```python
from build123d import *

# Parameters (mm, degrees)
SKETCH1_R           = 11.5
SKETCH1_R_2         = 1.75
BOSS_EXTRUDE1_DEPTH = 3.2
BOSS_EXTRUDE2_START = 3.2
SKETCH1_5_R         = 2.55
SKETCH1_5_R_2       = 11.5
SKETCH1_5_R_3       = 1.75
BOSS_EXTRUDE2_DEPTH = 3
BOSS_EXTRUDE3_START = 5
SKETCH1_6_R         = 2.55
BOSS_EXTRUDE3_DEPTH = 1.2
CUT_EXTRUDE2_START  = 3.2
SKETCH1_4_R         = 3
CUT_EXTRUDE2_DEPTH  = 3
FILLET1_R           = 3


with BuildPart() as part:
    # Sketch1 → Boss-Extrude1 (new body)
    with BuildSketch(Plane(origin=(0, -68.726755499, 0), x_dir=(1, 0, 0), z_dir=(0, 1, 0))):
        with BuildLine():
            Line((100.657671875, -32.65), (132.000817625, -32.65))
            ThreePointArc((132.000817625, -32.65), (132.689647804, -32.512983159), (133.273609832, -32.122792206))
            Line((133.273609832, -32.122792206), (136.602036956, -28.794365081))
            ThreePointArc((136.602036956, -28.794365081), (136.992227909, -28.210403054), (137.12924475, -27.521572875))
            Line((137.12924475, -27.521572875), (137.12924475, 3.821572875))
            ThreePointArc((137.12924475, 3.821572875), (136.992227909, 4.510403054), (136.602036956, 5.094365081))
            Line((136.602036956, 5.094365081), (133.273609832, 8.422792206))
            ThreePointArc((133.273609832, 8.422792206), (132.689647804, 8.812983159), (132.000817625, 8.95))
            Line((132.000817625, 8.95), (100.657671875, 8.95))
            ThreePointArc((100.657671875, 8.95), (99.968841697, 8.812983159), (99.384879669, 8.422792206))
            Line((99.384879669, 8.422792206), (96.056452544, 5.094365081))
            ThreePointArc((96.056452544, 5.094365081), (95.666261592, 4.510403054), (95.52924475, 3.821572875))
            Line((95.52924475, 3.821572875), (95.52924475, -27.521572875))
            ThreePointArc((95.52924475, -27.521572875), (95.666261592, -28.210403054), (96.056452544, -28.794365081))
            Line((96.056452544, -28.794365081), (99.384879669, -32.122792206))
            ThreePointArc((99.384879669, -32.122792206), (99.968841697, -32.512983159), (100.657671875, -32.65))
        make_face()
        with Locations((116.32924475, -11.85)):
            Circle(SKETCH1_R, mode=Mode.SUBTRACT)
        with Locations((100.82924475, -27.35)):
            Circle(SKETCH1_R_2, mode=Mode.SUBTRACT)
        with Locations((100.82924475, 3.65)):
            Circle(SKETCH1_R_2, mode=Mode.SUBTRACT)
        with Locations((131.82924475, 3.65)):
            Circle(SKETCH1_R_2, mode=Mode.SUBTRACT)
        with Locations((131.82924475, -27.35)):
            Circle(SKETCH1_R_2, mode=Mode.SUBTRACT)
    extrude(amount=BOSS_EXTRUDE1_DEPTH)

    # Sketch1<5> → Boss-Extrude2 (add)
    with BuildSketch(Plane(origin=(0, -68.726755499, 0), x_dir=(1, 0, 0), z_dir=(0, 1, 0)).offset(BOSS_EXTRUDE2_START)):
        with BuildLine():
            Line((108.32924475, 8.95), (100.657671875, 8.95))
            ThreePointArc((100.657671875, 8.95), (99.968841697, 8.812983159), (99.384879669, 8.422792206))
            Line((99.384879669, 8.422792206), (96.056452544, 5.094365081))
            ThreePointArc((96.056452544, 5.094365081), (95.666261592, 4.510403054), (95.52924475, 3.821572875))
            Line((95.52924475, 3.821572875), (95.52924475, -27.521572875))
            ThreePointArc((95.52924475, -27.521572875), (95.666261592, -28.210403054), (96.056452544, -28.794365081))
            Line((96.056452544, -28.794365081), (99.384879669, -32.122792206))
            ThreePointArc((99.384879669, -32.122792206), (99.968841697, -32.512983159), (100.657671875, -32.65))
            Line((100.657671875, -32.65), (156.32924475, -32.65))
            Line((156.32924475, -32.65), (156.32924475, 28))
            Line((156.32924475, 28), (108.32924475, 28))
            Line((108.32924475, 28), (108.32924475, 8.95))
        make_face()
        with Locations((144.32924475, -16)):
            Circle(SKETCH1_5_R, mode=Mode.SUBTRACT)
        with Locations((152.32924475, -16)):
            Circle(SKETCH1_5_R, mode=Mode.SUBTRACT)
        with Locations((144.32924475, -8)):
            Circle(SKETCH1_5_R, mode=Mode.SUBTRACT)
        with Locations((152.32924475, -8)):
            Circle(SKETCH1_5_R, mode=Mode.SUBTRACT)
        with Locations((120.32924475, 16)):
            Circle(SKETCH1_5_R, mode=Mode.SUBTRACT)
        with Locations((120.32924475, 24)):
            Circle(SKETCH1_5_R, mode=Mode.SUBTRACT)
        with Locations((144.32924475, 0)):
            Circle(SKETCH1_5_R, mode=Mode.SUBTRACT)
        with Locations((152.32924475, 0)):
            Circle(SKETCH1_5_R, mode=Mode.SUBTRACT)
        with Locations((144.32924475, 8)):
            Circle(SKETCH1_5_R, mode=Mode.SUBTRACT)
        with Locations((152.32924475, 8)):
            Circle(SKETCH1_5_R, mode=Mode.SUBTRACT)
        with Locations((128.32924475, 16)):
            Circle(SKETCH1_5_R, mode=Mode.SUBTRACT)
        with Locations((136.32924475, 16)):
            Circle(SKETCH1_5_R, mode=Mode.SUBTRACT)
        with Locations((128.32924475, 24)):
            Circle(SKETCH1_5_R, mode=Mode.SUBTRACT)
        with Locations((136.32924475, 24)):
            Circle(SKETCH1_5_R, mode=Mode.SUBTRACT)
        with Locations((144.32924475, 16)):
            Circle(SKETCH1_5_R, mode=Mode.SUBTRACT)
        with Locations((152.32924475, 16)):
            Circle(SKETCH1_5_R, mode=Mode.SUBTRACT)
        with Locations((144.32924475, 24)):
            Circle(SKETCH1_5_R, mode=Mode.SUBTRACT)
        with Locations((152.32924475, 24)):
            Circle(SKETCH1_5_R, mode=Mode.SUBTRACT)
        with Locations((116.32924475, -11.85)):
            Circle(SKETCH1_5_R_2, mode=Mode.SUBTRACT)
        with Locations((112.32924475, 24)):
            Circle(SKETCH1_5_R, mode=Mode.SUBTRACT)
        with Locations((112.32924475, 16)):
            Circle(SKETCH1_5_R, mode=Mode.SUBTRACT)
        with Locations((100.82924475, -27.35)):
            Circle(SKETCH1_5_R_3, mode=Mode.SUBTRACT)
        with Locations((100.82924475, 3.65)):
            Circle(SKETCH1_5_R_3, mode=Mode.SUBTRACT)
        with Locations((131.82924475, 3.65)):
            Circle(SKETCH1_5_R_3, mode=Mode.SUBTRACT)
        with Locations((131.82924475, -27.35)):
            Circle(SKETCH1_5_R_3, mode=Mode.SUBTRACT)
    extrude(amount=BOSS_EXTRUDE2_DEPTH)

    # Sketch1<6> → Boss-Extrude3 (add)
    with BuildSketch(Plane(origin=(0, -68.726755499, 0), x_dir=(1, 0, 0), z_dir=(0, 1, 0)).offset(BOSS_EXTRUDE3_START)):
        with Locations((152.32924475, -16)):
            Circle(SKETCH1_6_R)
        with Locations((144.32924475, -16)):
            Circle(SKETCH1_6_R)
        with Locations((144.32924475, -8)):
            Circle(SKETCH1_6_R)
        with Locations((152.32924475, -8)):
            Circle(SKETCH1_6_R)
        with Locations((152.32924475, 0)):
            Circle(SKETCH1_6_R)
        with Locations((144.32924475, 0)):
            Circle(SKETCH1_6_R)
        with Locations((152.32924475, 8)):
            Circle(SKETCH1_6_R)
        with Locations((152.32924475, 16)):
            Circle(SKETCH1_6_R)
        with Locations((144.32924475, 24)):
            Circle(SKETCH1_6_R)
        with Locations((152.32924475, 24)):
            Circle(SKETCH1_6_R)
        with Locations((136.32924475, 24)):
            Circle(SKETCH1_6_R)
        with Locations((136.32924475, 16)):
            Circle(SKETCH1_6_R)
        with Locations((128.32924475, 16)):
            Circle(SKETCH1_6_R)
        with Locations((128.32924475, 24)):
            Circle(SKETCH1_6_R)
        with Locations((120.32924475, 16)):
            Circle(SKETCH1_6_R)
        with Locations((120.32924475, 24)):
            Circle(SKETCH1_6_R)
        with Locations((144.32924475, 8)):
            Circle(SKETCH1_6_R)
        with Locations((144.32924475, 16)):
            Circle(SKETCH1_6_R)
        with Locations((112.32924475, 24)):
            Circle(SKETCH1_6_R)
        with Locations((112.32924475, 16)):
            Circle(SKETCH1_6_R)
    extrude(amount=BOSS_EXTRUDE3_DEPTH)

    # Sketch1<4> → Cut-Extrude2 (cut)
    with BuildSketch(Plane(origin=(0, -68.726755499, 0), x_dir=(1, 0, 0), z_dir=(0, 1, 0)).offset(CUT_EXTRUDE2_START)):
        with Locations((100.82924475, -27.35)):
            Circle(SKETCH1_4_R)
        with Locations((100.82924475, 3.65)):
            Circle(SKETCH1_4_R)
        with Locations((131.82924475, 3.65)):
            Circle(SKETCH1_4_R)
        with Locations((131.82924475, -27.35)):
            Circle(SKETCH1_4_R)
    extrude(amount=CUT_EXTRUDE2_DEPTH, mode=Mode.SUBTRACT)

    # Fillet1
    fillet1_edges = [part.edges().sort_by_distance(p)[0] for p in [
        (156.32924475, -64.026755499, 32.65),
        (108.32924475, -64.026755499, -8.95),
    ]]
    fillet(fillet1_edges, radius=FILLET1_R)


solid = part.part
```
Work out the finished part from the listing and answer in its coordinate system (mm). A direction names the side the tool comes from. Give positions to 0.01 mm unless a question says otherwise; leave off trailing zeros. Order: outer loops, then holes, each group sorted by start corner. A loop starts at its lowest first (then second) coordinate and runs counter-clockwise, first axis right, second up. Notation, with made-up numbers: (-13.5, -22) -> (33.5, -22) arc R37 ccw to (33.5, 14) -> close; hole circle Ø9 at (81, -2.5). An arc over 180 degrees is marked (long way). Answer as CSV lines item,"result". Start each with the question number.
(1) Section C-C, the plane x = 113.5 is taken. Write down the section's boundary in (y, z).
(2) Section B-B, the plane y = -67 is taken. Write down the section's boundary in (x, z).
(3) Consider line 1 along X through (y, z) = (-64.25, -9.5); line 2 along X through (y, z) = (-67, -4); line 3 along Y through (x, z) = (102, -2). Determine where each line is inside the solid, lowest interval first.
(4) Which of the six approach directions +Z, -Z, +X, -X, +Y, -Y give full straight-line access (tool end or side, diameter ignored) to faces 5 (the cylindrical face through (130.441, -67.149, 28.415)), 6 (the flat face through (144, -63.727, 16)), 7 (the flat face through (102, -65.527, -2))?
(5) Section A-A, the plane z = 11.85 is taken. Write down the section's boundary in (x, y), plus the area to 3 significant figures.
(6) Section D-D, the plane z = -24 is taken. Write down the section's boundary in (x, y).
(7) Each of these flat-tipped pins is pushed along its axis until it touches: pin 1 Ø5.5 at (x, z) = (136.5, -23) entering from -Y; pin 2 Ø2.5 at (x, z) = (144.5, 7) entering from -Y; pin 3 Ø1 at (x, y) = (102, -66.5) entering from -Z. Where does it stop, or does it pass through?
(8) For a pull along Z with two mould halves and no side action, classify faces 1 (the flat face through (121, -65, 32.65)), 2 (the flat face through (95.529, -66, 12)), 3 (the flat face through (133, -65.527, 29)), 4 (the cylindrical face through (109.78, -64.64, -16.11)) as released by +Z, released by -Z, zero draft, split by the parting line, or undercut.
Entries:
1,outline,"(-68.73, -8.95) -> (-65.53, -8.95) -> (-65.53, -13.73) -> (-63.73, -13.73) -> (-63.73, -18.27) -> (-65.53, -18.27) -> (-65.53, -21.73) -> (-63.73, -21.73) -> (-63.73, -26.27) -> (-65.53, -26.27) -> (-65.53, -28) -> (-62.53, -28) -> (-62.53, 0.7) -> (-68.73, 0.7) -> close; (-68.73, 23) -> (-62.53, 23) -> (-62.53, 32.65) -> (-68.73, 32.65) -> close"
2,outline,"(95.53, -3.82) arc R1.8 ccw to (96.06, -5.09) -> (99.38, -8.42) arc R1.8 ccw to (100.66, -8.95) -> (132, -8.95) arc R1.8 ccw to (133.27, -8.42) -> (136.6, -5.09) arc R1.8 ccw to (137.13, -3.82) -> (137.13, 27.52) arc R1.8 ccw to (136.6, 28.79) -> (133.27, 32.12) arc R1.8 ccw to (132, 32.65) -> (100.66, 32.65) arc R1.8 ccw to (99.38, 32.12) -> (96.06, 28.79) arc R1.8 ccw to (95.53, 27.52) -> close; hole circle Ø3.5 at (100.83, -3.65); hole circle Ø3.5 at (100.83, 27.35); hole circle Ø23 at (116.33, 11.85); hole circle Ø3.5 at (131.83, -3.65); hole circle Ø3.5 at (131.83, 27.35)"
3,line 1,"107.06 to 142.27, 146.39 to 150.27, 154.39 to 156.33"
3,line 2,"95.54 to 99.11, 102.54 to 130.11, 133.54 to 137.12"
3,line 3,"-68.73 to -65.53"
4,face 5,"+Y, -Y"
4,face 6,"-Y"
4,face 7,"+Y"
5,outline,"(95.53, -68.73) -> (104.83, -68.73) -> (104.83, -62.53) -> (95.53, -62.53) -> close; (127.83, -68.73) -> (137.13, -68.73) -> (137.13, -65.53) -> (156.33, -65.53) -> (156.33, -62.53) -> (127.83, -62.53) -> close"
5,area,"173 mm²"
6,outline,"(108.33, -65.53) -> (109.78, -65.53) -> (109.78, -63.73) -> (114.88, -63.73) -> (114.88, -65.53) -> (117.78, -65.53) -> (117.78, -63.73) -> (122.88, -63.73) -> (122.88, -65.53) -> (125.78, -65.53) -> (125.78, -63.73) -> (130.88, -63.73) -> (130.88, -65.53) -> (133.78, -65.53) -> (133.78, -63.73) -> (138.88, -63.73) -> (138.88, -65.53) -> (141.78, -65.53) -> (141.78, -63.73) -> (146.88, -63.73) -> (146.88, -65.53) -> (149.78, -65.53) -> (149.78, -63.73) -> (154.88, -63.73) -> (154.88, -65.53) -> (156.33, -65.53) -> (156.33, -62.53) -> (108.33, -62.53) -> close"
7,pin 1,"y = -65.53"
7,pin 2,"y = -63.73"
7,pin 3,"z = -8.95"
8,face 1,"released by +Z"
8,face 2,"zero draft"
8,face 3,"undercut"
8,face 4,"undercut"
